Geometry: see drawing. Coordinates: mm, zero at the bounding-box minimum. A direction names the side the tool comes from. Round coordinates to 2 decimals unless told otherwise and drop trailing zeros. Write each loop counter-clockwise with the first axis right and the second up, starting at its lowest first coordinate (ties: lowest second). Pieces come first, ordered by that corner, then holes.
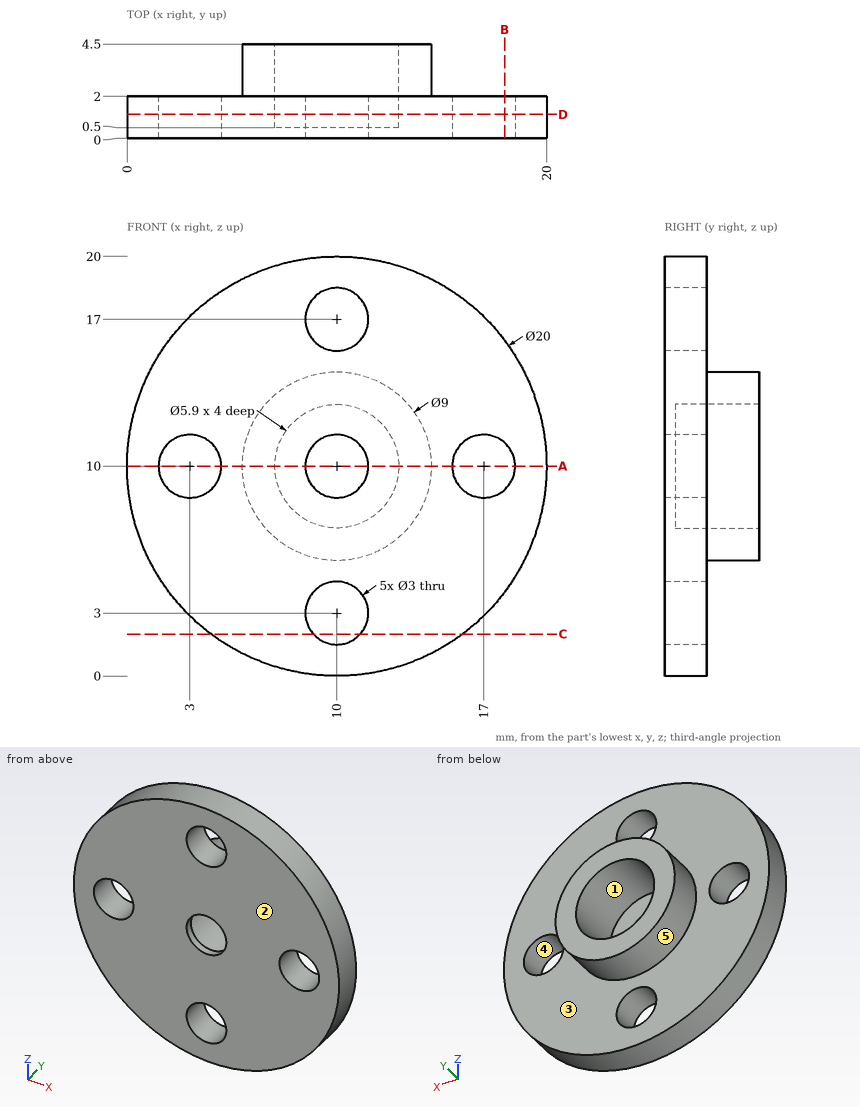
1) Pull-direction query (Z, two-part tool) for the marked faces 3, 4 and 5; classes: released by +Z, released by -Z, zero draft, split by the parting line, or undercut.
Taken from the geometry:
face 3: zero draft
face 4: undercut
face 5: split by the parting line
2) Material intervals for line 1 (X direction, y = 0.3, z = 10); line 2 (X direction, y = 0.55, z = 10.5); line 3 (Y direction, x = 6.25, z = 16.25), sorted ascending.
Taken from the geometry:
line 1: x = 0 to 1.5, 4.5 to 8.5, 11.5 to 15.5, 18.5 to 20
line 2: x = 0.01 to 1.59, 4.41 to 7.09, 12.91 to 15.59, 18.41 to 19.99
line 3: y = 0 to 2
3) Section query B-B on x = 18. Return the cut outline in (y, z).
Taken from the geometry:
outline: (0, 4) - (2, 4) - (2, 8.88) - (0, 8.88) - close; (0, 11.12) - (2, 11.12) - (2, 16) - (0, 16) - close
4) Reachability of the marked faces 1 and 2 from +Z, -Z, +X, -X, +Y, -Y: full face, straight path, thin tool, end or side. Return the list, or none.
Taken from the geometry:
face 1: +Y
face 2: +Z, -Z, +X, -X, -Y
5) Contact query for a flat-ended pin moving along its axis: P1, Ø2.5, axis at x = 17, z = 10, coming from the -Y side. Output: stop coordinate, or through.
Taken from the geometry:
P1: passes through
6) Section query C-C on z = 2. Return the cut outline in (x, y).
Taken from the geometry:
outline: (4, 0) - (8.88, 0) - (8.88, 2) - (4, 2) - close; (11.12, 0) - (16, 0) - (16, 2) - (11.12, 2) - close
7) Section query A-A on z = 10. Return the cut outline in (x, y).
Taken from the geometry:
outline: (0, 0) - (1.5, 0) - (1.5, 2) - (0, 2) - close; (4.5, 0) - (8.5, 0) - (8.5, 0.5) - (7.05, 0.5) - (7.05, 4.5) - (5.5, 4.5) - (5.5, 2) - (4.5, 2) - close; (11.5, 0) - (15.5, 0) - (15.5, 2) - (14.5, 2) - (14.5, 4.5) - (12.95, 4.5) - (12.95, 0.5) - (11.5, 0.5) - close; (18.5, 0) - (20, 0) - (20, 2) - (18.5, 2) - close
8) Section query D-D on y = 1.15. Return the cut outline in (x, z), then the cut area to 3 significant figures.
Taken from the geometry:
outline: circle Ø20 at (10, 10); hole circle Ø3 at (3, 10); hole circle Ø5.9 at (10, 10); hole circle Ø3 at (10, 3); hole circle Ø3 at (10, 17); hole circle Ø3 at (17, 10)
area: 259 mm2
